Here's how the part is built. I have some questions about the finished solid (model axes, mm). A direction names the side the tool comes from. Round coordinates to 2 decimals unless told otherwise and drop trailing zeros. Order: outer loops, then holes, each group sorted by start corner. A loop starts at its lowest first (then second) coordinate and runs counter-clockwise, first axis right, second up.
Autodesk Inventor part; units mm, degrees
ref_plane "YZ Plane" through (0, 0, 0) normal (1, 0, 0) x (0, 1, 0)
ref_plane "XZ Plane" through (0, 0, 0) normal (0, 1, 0) x (-1, 0, 0)
ref_plane "XY Plane" through (0, 0, 0) normal (0, 0, 1) x (1, 0, 0)
sketch "Sketch1" plane through (0, 0, 0) normal (0, 0, 1) x (1, 0, 0)
  circle A0 centre (0, 0) radius 3
  dimension "d0" = 6
extrude "Extrusion1" add sketch "Sketch1" along normal blind 120
thread "Thread1"
chamfer "Chamfer1" distance 0.6 angle 45 1 edges at (-3, 0, 120)
chamfer "Chamfer2" distance 0.6 angle 45 1 edges at (-3, 0, 0)
sketch "Sketch2" plane through (0, 0, 120) normal (0, 0, 1) x (1, 0, 0)
  line L0 (3.8696, 4.6025) -> (-3.8038, 4.6025)
  line L1 (-3.8038, 4.6025) -> (-3.8038, 2)
  line L2 (-3.8038, 2) -> (3.8696, 2)
  line L3 (3.8696, 2) -> (3.8696, 4.6025)
  point P0 (0, 0)
  dimension "d11" = 2
extrude "Extrusion2" cut sketch "Sketch2" against normal blind 8
properties part number "popychacz"
1) I'm going to push flat-ended pins straight in: pin 1 (3 mm diameter, centred on x = -0.5, y = 0, fed in from -Z); pin 2 (1.5 mm diameter, centred on x = 1, z = 32.5, fed in from -Y); pin 3 (2 mm diameter, centred on x = 0.5, z = 116, fed in from +Y); pin 4 (0.5 mm diameter, centred on x = -1, y = 2.5, fed in from +Z). Where does each tip first touch, or does it pass through?
2) If we section it at A-A (z = 96): Write out the boundary of the cut face in (x, y), plus the area to 3 significant figures.
3) For faces 1 (the flat face through (0, 2, 116)), 2 (the cylindrical face through (-3, 0, 59)), which set-ups out of +Z, -Z, +X, -X, +Y, -Y let a thin tool reach every point of the face, with its end or its side?
4) I need wall thicknesses on line 1 (Y direction, x = -0.2, z = 87); line 2 (X direction, y = 2, z = 49.5). Which ranges of each line are inside material? Lowest first, please.
Solutions:
1. pin 1: stops at z = 0
1. pin 2: stops at y = -2.99
1. pin 3: stops at y = 2
1. pin 4: stops at z = 112
2. outline: circle Ø6 at (0, 0)
2. area: 28.3 mm2
3. face 1: +Z, +X, -X, +Y
3. face 2: +Z, -Z
4. line 1: y = -2.99 to 2.99
4. line 2: x = -2.24 to 2.24
